from build123d import *

# Parameters (mm, degrees)
BOSS_EXTRUDE1_DEPTH = 9
SKETCH2_W           = 14
SKETCH2_H           = 1225
CUT_EXTRUDE1_DEPTH  = 10
SKETCH3_W           = 82
SKETCH3_H           = 82
CUT_EXTRUDE5_DEPTH  = 10
SKETCH4_R           = 2.75
CUT_EXTRUDE6_DEPTH  = 10


with BuildPart() as part:
    # Sketch1 → Boss-Extrude1 (new body)
    with BuildSketch(Plane(origin=(0, 0, 0), x_dir=(1, 0, 0), z_dir=(0, 1, 0))):
        Polygon((-304.5, -532.5), (-304.5, -612.5), (224.5, -612.5), (304.5, -612.5), (304.5, -532.5), (304.5, 497.5), (304.5, 612.5), (224.5, 612.5), (-304.5, 612.5), (-304.5, 497.5), align=None)
    extrude(amount=BOSS_EXTRUDE1_DEPTH)

    # Sketch2 → Cut-Extrude1 (cut)
    with BuildSketch(Plane(origin=(0, 9, 0), x_dir=(1, 0, 0), z_dir=(0, 1, 0))):
        with Locations((297.5, 0)):
            Rectangle(SKETCH2_W, SKETCH2_H)
    extrude(amount=-CUT_EXTRUDE1_DEPTH, mode=Mode.SUBTRACT)

    # Sketch3 → Cut-Extrude5 (cut)
    with BuildSketch(Plane(origin=(0, 9, 0), x_dir=(1, 0, 0), z_dir=(0, 1, 0))):
        with Locations((-263.5, 571.5)):
            Rectangle(SKETCH3_W, SKETCH3_H)
        with Locations((-263.5, -571.5)):
            Rectangle(SKETCH3_W, SKETCH3_H)
    extrude(amount=-CUT_EXTRUDE5_DEPTH, mode=Mode.SUBTRACT)

    # Sketch4 → Cut-Extrude6 (cut)
    with BuildSketch(Plane(origin=(0, 9, 0), x_dir=(1, 0, 0), z_dir=(0, 1, 0))):
        with Locations(Location((23, 47.631397208, 0), (0, 0, 270))):
            Circle(SKETCH4_R)
        with Locations(Location((-32, -47.631397208, 0), (0, 0, 270))):
            Circle(SKETCH4_R)
        with Locations(Location((23, -47.631397208, 0), (0, 0, 270))):
            Circle(SKETCH4_R)
        with Locations(Location((50.5, 0, 0), (0, 0, 270))):
            Circle(SKETCH4_R)
        with Locations(Location((-32, 47.631397208, 0), (0, 0, 270))):
            Circle(SKETCH4_R)
    extrude(amount=-CUT_EXTRUDE6_DEPTH, mode=Mode.SUBTRACT)


solid = part.part
Work out the finished part from the listing and answer in its coordinate system (mm). Coordinates: 2 decimals unless noted, no trailing zeros. Write each loop counter-clockwise with the first axis right and the second up, starting at its lowest first coordinate (ties: lowest second). Pieces come first, ordered by that corner, then holes.
1. Consider line 1 along X through (y, z) = (4.5, 0); line 2 along X through (y, z) = (0.5, -541). Determine where each line is inside the solid, lowest interval first.
Results list:
line 1: x = -304.5 to 47.75, 53.25 to 290.5
line 2: x = -222.5 to 290.5
2. The part is cut by section A-A, the plane y = 5.5. Write down the section's boundary in (x, z), and give its area (3 significant figures).
Results list:
outline: (-304.5, -530.5) - (-222.5, -530.5) - (-222.5, -612.5) - (290.5, -612.5) - (290.5, 612.5) - (-222.5, 612.5) - (-222.5, 530.5) - (-304.5, 530.5) - close; hole circle Ø5.5 at (-32, -47.63); hole circle Ø5.5 at (-32, 47.63); hole circle Ø5.5 at (23, -47.63); hole circle Ø5.5 at (23, 47.63); hole circle Ø5.5 at (50.5, 0)
area: 715,000 mm2
3. A flat-ended cylindrical pin translates along its axis: pin 1 (4.5 mm diameter, centred on x = 50.5, z = 0, fed in from +Y). Find the tip coordinate at first contact, or state that the pin passes through.
Results list:
pin 1: passes through
